CAD build for the part. Positions are in the model's coordinates, mm. A direction names the side the tool comes from. Give positions to 0.01 mm unless a question says otherwise; leave off trailing zeros. Loops run counter-clockwise (first coordinate to the right, second up) from the corner with the lowest first, then second, coordinate; pieces in that order, holes last. Notation, with made-up numbers: (57.25, -14.75) -> (78.25, -14.75) arc R18 ccw to (78.25, 19.25) -> close; hole circle Ø4 at (40.25, 83.25). An arc over 180 degrees is marked (long way). Use one line per item in the form item = value.
Autodesk Fusion 360 part; units mm, degrees
sketch "スケッチ1" plane through (0, 0, 0) normal (0, 0, 1) x (1, 0, 0)
  line L0 (-17.5, 11) -> (17.5, 11)
  line L1 (17.5, 11) -> (17.5, 0)
  line L2 (17.5, 0) -> (-17.5, 0)
  line L3 (-17.5, 0) -> (-17.5, 11)
  dimension "d1" = 35
  dimension "d2" = 11
extrude "押し出し1" add sketch "スケッチ1" along normal blind 120
sketch "スケッチ2" plane through (0, 0, 0) normal (0, 0, -1) x (1, 0, 0)
  line L0 (17.5, 0) -> (-17.5, 0)
  line L1 (-17.5, 0) -> (-17.5, -11)
  line L2 (-17.5, -11) -> (17.5, -11)
  line L3 (17.5, -11) -> (17.5, 0)
  circle A0 centre (0, 0) radius 3.4
  dimension "d5" = 6.8
extrude "押し出し2" cut sketch "スケッチ2" against normal blind 20 contours L0 A0 picked at (0.8532, -1.8586)
sketch "スケッチ3" plane through (0, 0, 120) normal (0, 0, 1) x (-1, 0, 0)
  line L0 (17.5, 0) -> (-17.5, 0)
  line L1 (-17.5, 0) -> (-17.5, -11)
  line L2 (-17.5, -11) -> (17.5, -11)
  line L3 (17.5, -11) -> (17.5, 0)
  line L4 (15.5, -9) -> (-15.5, -9)
  line L5 (-15.5, -9) -> (-15.5, 0)
  line L6 (-15.5, 0) -> (15.5, 0)
  line L7 (15.5, 0) -> (15.5, -9)
  dimension "d8" = 2
  dimension "d9" = 31
extrude "押し出し3" cut sketch "スケッチ3" against normal blind 100 contours L0 L4 L5 L6 L7
ref_plane "作業平面1" through (0, 5.5, 9) normal (0, 0, -1) x (-1, 0, 0)
sketch "スケッチ5" plane through (0, 11, 0) normal (0, 1, 0) x (-1, 0, 0)
  line L0 (-17.5, 0) -> (17.5, 0)
  line L1 (17.5, 0) -> (17.5, 120)
  line L2 (17.5, 120) -> (-17.5, 120)
  line L3 (-17.5, 120) -> (-17.5, 0)
  line L4 (-17.5, 130) -> (17.5, 130)
  line L5 (17.5, 130) -> (17.5, 120)
  line L6 (17.5, 120) -> (-17.5, 120)
  line L7 (-17.5, 120) -> (-17.5, 130)
  line L8 (-17.5, 125) -> (17.5, 125) construction
  circle A0 centre (12, 125) radius 2
  circle A1 centre (-12, 125) radius 2
  dimension "d16" = 4
  dimension "d17" = 4
  dimension "d18" = 24
  dimension "d19" = 10
  dimension "d20" = 5.5
extrude "押し出し5" add sketch "スケッチ5" against normal blind 2 contours L2 L4 L5 L6 L7
sketch "スケッチ8" plane through (0, 0, 0) normal (0, -1, 0) x (1, 0, 0)
  line L0 (-3.4, 20) -> (-15.5, 20)
  line L1 (-15.5, 20) -> (-15.5, 120)
  line L2 (-15.5, 120) -> (-17.5, 120)
  line L3 (-17.5, 120) -> (-17.5, 0)
  line L4 (-17.5, 0) -> (-3.4, 0)
  line L5 (-3.4, 0) -> (-3.4, 20)
  circle A0 centre (-14, 15) radius 2.55
  line L6 (18.5, 15) -> (-17.5, 15) construction
  line L7 (17.541, 5) -> (-17.5, 5) construction
  line L8 (15.5, 20) -> (3.4, 20) construction
  circle A1 centre (14, 15) radius 2.55
  circle A2 centre (14, 5) radius 2.55
  circle A3 centre (-14, 5) radius 2.55
  line L9 (17.5, 0) -> (17.5, 120)
  dimension "d30" = 5
  dimension "d31" = 10
  dimension "d32" = 5.1
  dimension "d33" = 5.1
  dimension "d34" = 5.1
  dimension "d35" = 5.1
  dimension "d36" = 3.5
  dimension "d37" = 3.5
  dimension "d38" = 3.5
  dimension "d39" = 3.5
extrude "押し出し8" cut sketch "スケッチ8" against normal blind 15 contours A0 | A1 | A2 | A3
move_face "OffsetFaces1" offset 3 1 faces at (-3.8517, 11, 52.6741)
sketch "Sketch9" plane through (0, 9, 0) normal (0, -1, 0) x (1, 0, 0)
  circle A0 centre (12, 125) radius 2
  circle A1 centre (-12, 125) radius 2
  line L0 (-15.5, 120) -> (-15.5, 20)
  line L1 (-15.5, 20) -> (15.5, 20)
  line L2 (15.5, 20) -> (15.5, 120)
  line L3 (15.5, 120) -> (17.5, 120)
  line L4 (17.5, 120) -> (17.5, 130)
  line L5 (17.5, 130) -> (-17.5, 130)
  line L6 (-17.5, 130) -> (-17.5, 120)
  line L7 (-17.5, 120) -> (-15.5, 120)
  point P0 (12.5, 50)
  point P1 (-12.5, 50)
  point P2 (-12.5, 92)
  point P3 (12.5, 92)
hole "Hole1" at (-12.5, 9, 92) at (12.5, 9, 92) at (12.5, 9, 50) at (-12.5, 9, 50) direction (0, 1, 0) diameter 3.4 depth 9 tip angle 118 countersink diameter 5.6 countersink angle 90
ref_plane "WorkPlane2" through (0, 0, 17) normal (0, 0, 1) x (1, 0, 0)
sketch "Sketch10" plane through (0, 0, 17) normal (0, 0, 1) x (1, 0, 0)
  line L0 (0, 6) -> (9.5, 2.25)
  line L1 (9.5, 2.25) -> (9.5, 0)
  line L2 (0, 6) -> (-9.5, 2.25)
  line L3 (-9.5, 2.25) -> (-9.5, 0)
  line L4 (-9.5, 0) -> (9.5, 0)
extrude "Extrude9" cut sketch "Sketch10" along normal blind 0.65 and the other way blind 0.65
sketch "Sketch11" plane through (0, 9, 0) normal (0, -1, 0) x (1, 0, 0)
  circle A0 centre (12.5, 50) radius 2.8
  circle A1 centre (-12.5, 92) radius 2.8
  circle A2 centre (12.5, 92) radius 2.8
  circle A3 centre (-12.5, 50) radius 2.8
  circle A4 centre (-12, 125) radius 2
  circle A5 centre (12, 125) radius 2
  line L0 (-15.5, 120) -> (-15.5, 20)
  line L1 (-15.5, 20) -> (15.5, 20)
  line L2 (15.5, 20) -> (15.5, 120)
  line L3 (15.5, 120) -> (17.5, 120)
  line L4 (17.5, 120) -> (17.5, 130)
  line L5 (17.5, 130) -> (-17.5, 130)
  line L6 (-17.5, 130) -> (-17.5, 120)
  line L7 (-17.5, 120) -> (-15.5, 120)
  line L8 (-17.5, 130) -> (17.5, 130)
  line L9 (17.5, 130) -> (17.5, 120)
  line L10 (17.5, 120) -> (-17.5, 120)
  line L11 (-17.5, 120) -> (-17.5, 130)
extrude "Extrude10" cut sketch "Sketch11" against normal blind 3 contours L3 L4 L5 L6 L7 L8 L9 L10 L11
move_face "OffsetFaces2" offset 2 1 faces at (-3.9094, 14, 64.5049)
move_face "OffsetFaces3" offset 15 1 faces at (5.8333, 13.3333, 130)
sketch "Sketch12" plane through (0, 12, 0) normal (0, -1, 0) x (1, 0, 0)
  circle A0 centre (12, 125) radius 2
  circle A1 centre (-12, 125) radius 2
  line L0 (-17.5, 120) -> (17.5, 120)
  line L1 (17.5, 120) -> (17.5, 145)
  line L2 (17.5, 145) -> (-17.5, 145)
  line L3 (-17.5, 145) -> (-17.5, 120)
  point P0 (-12, 140)
  point P1 (12, 140)
hole "Hole2" at (-12, 12, 140) at (12, 12, 140) direction (0, 1, 0) diameter 4 depth 5 tip angle 118
1. Cut at A-A, the plane z = 5. Write the cut outline in (x, y), then the cut area to 3 significant figures.
Result sheet:
outline = (-17.5, 0) -> (-16.55, 0) -> (-16.55, 16) -> (-17.5, 16) -> close; (-11.45, 0) -> (-3.4, 0) arc R3.4 cw to (3.4, 0) -> (11.45, 0) -> (11.45, 16) -> (-11.45, 16) -> close; (16.55, 0) -> (17.5, 0) -> (17.5, 16) -> (16.55, 16) -> close
area = 379 mm^2
2. Cut at B-B, the plane y = 7.25. Write the cut outline in (x, z).
Result sheet:
outline = (-17.5, 0) -> (17.5, 0) -> (17.5, 120) -> (15.5, 120) -> (15.5, 20) -> (-15.5, 20) -> (-15.5, 120) -> (-17.5, 120) -> close; hole circle Ø5.1 at (-14, 5); hole circle Ø5.1 at (-14, 15); hole circle Ø5.1 at (14, 5); hole circle Ø5.1 at (14, 15)
3. Drop flat-ended pins along their axis: P1, Ø3, axis at x = -1.5, y = 2, coming from the +Z side; P2, Ø1.8, axis at x = 1, y = 2.5, coming from the -Z side; P3, Ø4.5, axis at x = 12, z = 125, coming from the -Y side; P4, Ø6, axis at x = 6.5, z = 59, coming from the -Y side. Give the stop position or say it passes through.
Result sheet:
P1 = 20
P2 = 0
P3 = 12
P4 = 9
4. Cut at D-D, the plane x = -1.5. Write the cut outline in (y, z), then the cut area to 3 significant figures.
Result sheet:
outline = (3.05, 0) -> (16, 0) -> (16, 145) -> (12, 145) -> (12, 120) -> (9, 120) -> (9, 20) -> (3.05, 20) -> (3.05, 17.65) -> (5.41, 17.65) -> (5.41, 16.35) -> (3.05, 16.35) -> close
area = 1,060 mm^2
5. Drill centre lines: line 1 (Z direction, x = 14, y = 6.5); line 2 (X direction, y = 14.35, z = 50); line 3 (Z direction, x = 4.5, y = 3). Where is each one in solid material? Low to high.
Result sheet:
line_1 = 0 to 2.45, 7.55 to 12.45, 17.55 to 20
line_2 = -17.5 to -14.2, -10.8 to 10.8, 14.2 to 17.5
line_3 = 0 to 16.35, 17.65 to 20
6. Cut at C-C, the plane z = 34. Write the cut outline in (x, y).
Result sheet:
outline = (-17.5, 0) -> (-15.5, 0) -> (-15.5, 9) -> (15.5, 9) -> (15.5, 0) -> (17.5, 0) -> (17.5, 16) -> (-17.5, 16) -> close
7. Tool access for faces 1 (the cylindrical face through (-12, 14, 142)), 2 (the flat face through (0, 4, 20)), 3 (the flat face through (-1, 10, 120)), 4 (the flat face through (-4.683, 4.151, 16.991)): list every direction of +Z, -Z, +X, -X, +Y, -Y with a clear straight run to the whole face (end or side of a thin tool).
Result sheet:
face_1 = +Y, -Y
face_2 = +Z, -Y
face_3 = +Z, +X, -X, -Y
face_4 = -Y
8. Mould opens along X. For faces 5 (the cylindrical face through (12, 14, 142)), 6 (the flat face through (0, 12, 133)), 7 (the flat face through (0, 4, 17.65)), 8 (the flat face through (-17.5, 8, 57)) say: pulls with the +X half, pulls with the -X half, needs draft (parallel to the pull), parting line crosses it, or undercut.
Result sheet:
face_5 = undercut
face_6 = needs draft
face_7 = undercut
face_8 = pulls with the -X half
